```python
from build123d import *

# Parameters (mm, degrees)
F0_W     = 300
F0_H     = 200
F1_DEPTH = 250
F3_T     = -20
F4_D     = 150


with BuildPart() as f1:
    # F0 (on Top) → F1 (new body)
    with BuildSketch(Plane.XY):
        Rectangle(F0_W, F0_H)
    extrude(amount=F1_DEPTH)

    # F3
    f3_openings = [f1.faces().sort_by_distance(p)[0] for p in [
        (0, 0, 0),
    ]]
    offset(amount=F3_T, openings=f3_openings)

    # F4 (through all)
    with Locations(Plane.XY.offset(250)):
        with Locations((0, 0)):
            Hole(F4_D / 2)


solid = f1.part
```
Work out the finished part from the listing and answer in its coordinate system (mm). A direction names the side the tool comes from. Round coordinates to 2 decimals unless told otherwise and drop trailing zeros. Order: outer loops, then holes, each group sorted by start corner. A loop starts at its lowest first (then second) coordinate and runs counter-clockwise, first axis right, second up.
Q1. The mould has two halves that part along X. Classify faces 1 (the flat face through (-2, -100, 123)), 2 (the flat face through (-130, -1, 113)), 3 (the flat face through (150, -1, 123)): pulls with the +X half, pulls with the -X half, needs draft (parallel to the pull), parting line crosses it, or undercut.
Solution:
face 1: needs draft
face 2: undercut
face 3: pulls with the +X half
Q2. A cutting plane is placed at D-D, the plane x = 85. Determine the outline of the cut face in (y, z), then the cut area to 3 significant figures.
Solution:
outline: (-100, 0) - (-80, 0) - (-80, 230) - (80, 230) - (80, 0) - (100, 0) - (100, 250) - (-100, 250) - close
area: 13,200 mm2
Q3. A cutting plane is placed at B-B, the plane y = 0. Determine the outline of the cut face in (x, z), then the cut area to 3 significant figures.
Solution:
outline: (-150, 0) - (-130, 0) - (-130, 230) - (-75, 230) - (-75, 250) - (-150, 250) - close; (75, 230) - (130, 230) - (130, 0) - (150, 0) - (150, 250) - (75, 250) - close
area: 12,200 mm2
Q4. A tool of negligible diameter and unlimited length cuts with its end or side. For faces 4 (the flat face through (-35, 68, 250)), 5 (the flat face through (130, -1, 113)), from which of +Z, -Z, +X, -X, +Y, -Y can it reach the whole face along a straight path? Write none if from no direction.
Solution:
face 4: +Z, +X, -X, +Y, -Y
face 5: -Z
Q5. A cutting plane is placed at C-C, the plane z = 56. Determine the outline of the cut face in (x, y).
Solution:
outline: (-150, -100) - (150, -100) - (150, 100) - (-150, 100) - close; hole (-130, -80) - (130, -80) - (130, 80) - (-130, 80) - close
Q6. Find the intervals of material crossed by line 1 along X through (y, z) = (-67, 96.5); line 2 along Y through (x, z) = (-63, 61.5); line 3 along Y through (x, z) = (0, 239), in increasing order.
Solution:
line 1: x = -150 to -130, 130 to 150
line 2: y = -100 to -80, 80 to 100
line 3: y = -100 to -75, 75 to 100
Q7. A cutting plane is placed at A-A, the plane x = 0. Determine the outline of the cut face in (y, z).
Solution:
outline: (-100, 0) - (-80, 0) - (-80, 230) - (-75, 230) - (-75, 250) - (-100, 250) - close; (75, 230) - (80, 230) - (80, 0) - (100, 0) - (100, 250) - (75, 250) - close
Q8. Given pin 1 Ø4 at (x, y) = (-86.5, -44) entering from -Z, flat-ended and moving along its own axis, determine where the tip first touches the part or whether it passes through.
Solution:
pin 1: stops at z = 230
